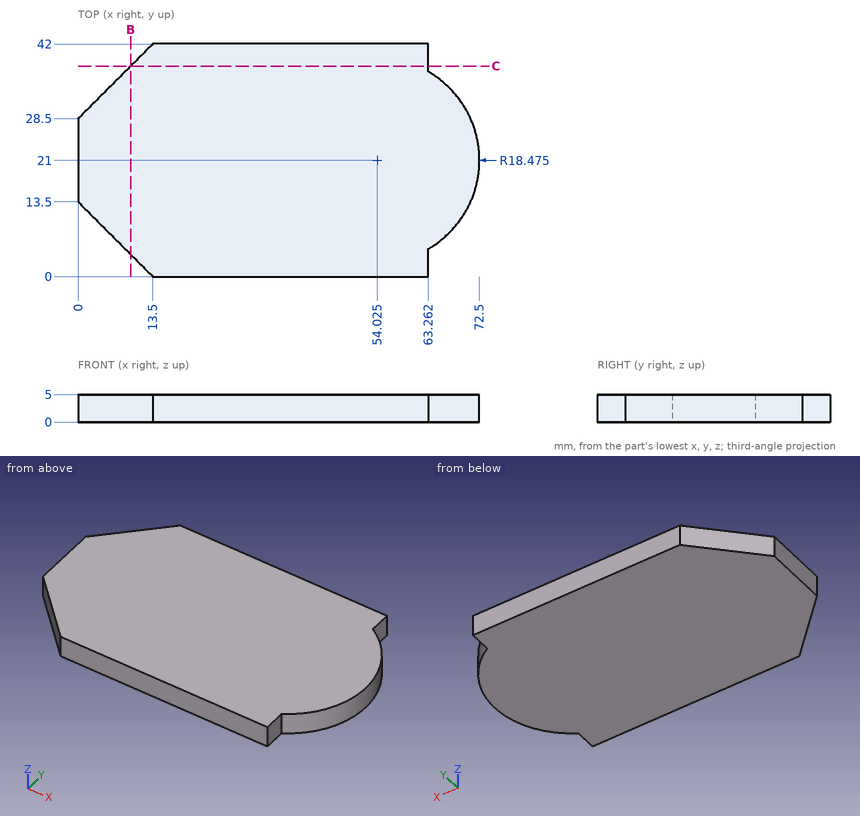
Design review of the part shown in the three views and the two pictorial views. Dimensions are in mm from the part's minimum x, y and z. Coordinates: 2 decimals unless noted, no trailing zeros. Order: outer loops, then holes, each group sorted by start corner. A loop starts at its lowest first (then second) coordinate and runs counter-clockwise, first axis right, second up. Notation, with made-up numbers: (64.5, -16) - (96.5, -16) arc R27 cw to (96.5, 3) - close; hole circle Ø5 at (-5, 71.25). An arc over 180 degrees is marked (long way). Answer as CSV lines item,"result". Start each with the question number.
1) Insertion check: P1, Ø1.5, axis at y = 3.5, z = 2, coming from the +X side. The pin has a flat end and moves straight along its axis. Give the tip position at first contact, or say it passes through.
2) Add section B-B (x = 9.5). State the section outline as (y, z) points, then the cut area to 3 significant figures.
3) Add section C-C (y = 38). State the section outline as (x, z) points.
4) To check wall thickness, follow line 1 along X through (y, z) = (3, 3.05); line 2 along X through (y, z) = (38, 0.5); line 3 along Y through (x, z) = (12.5, 1.5). State the ranges of each line that lie inside material, in increasing order. Write a range as [from, to].
Result:
1,P1,"x = 63.26"
2,outline,"(4, 0) - (38, 0) - (38, 5) - (4, 5) - close"
2,area,"170 mm^2"
3,outline,"(9.5, 0) - (63.26, 0) - (63.26, 5) - (9.5, 5) - close"
4,line 1,"[10.5, 63.26]"
4,line 2,"[9.5, 63.26]"
4,line 3,"[1, 41]"
